```python
from build123d import *

# Parameters (mm, degrees)
SKETCH1_R           = 100
BOSS_EXTRUDE1_DEPTH = 30
FILLET2_R           = 10
SKETCH2_R           = 20
SKETCH2_R_2         = 15
BOSS_EXTRUDE2_DEPTH = 50


with BuildPart() as part:
    # Sketch1 → Boss-Extrude1 (new body)
    with BuildSketch(Plane.XY):
        Circle(SKETCH1_R)
        with BuildLine():
            Line((-10.606601718, -10.606601718), (-49.497474683, -49.497474683))
            ThreePointArc((-49.497474683, -49.497474683), (-69.64553071, -7.03562734), (-58.396917549, 38.597927675))
            Line((-58.396917549, 38.597927675), (-10.606601718, -10.606601718))
        make_face(mode=Mode.SUBTRACT)
        with BuildLine():
            ThreePointArc((10.606601718, -10.606601718), (13.858192988, -5.740251485), (15, 0))
            Line((15, 0), (70, 0))
            ThreePointArc((70, 0), (33.601511791, -61.407966954), (-37.741097297, -58.954300732))
            Line((-37.741097297, -58.954300732), (10.606601718, -10.606601718))
        make_face(mode=Mode.SUBTRACT)
        with BuildLine():
            ThreePointArc((0, 15), (-5.740251485, 13.858192988), (-10.606601718, 10.606601718))
            Line((-10.606601718, 10.606601718), (-49.497474683, 49.497474683))
            ThreePointArc((-49.497474683, 49.497474683), (20.152118643, 67.036498374), (68.585712798, 14))
            Line((68.585712798, 14), (0, 15))
        make_face(mode=Mode.SUBTRACT)
    extrude(amount=BOSS_EXTRUDE1_DEPTH)

    # Fillet2
    fillet2_edges = [part.edges().sort_by_distance(p)[0] for p in [
        (-100, 0, 0),
        (-100, 0, 30),
    ]]
    fillet(fillet2_edges, radius=FILLET2_R)

    # Sketch2 → Boss-Extrude2 (add)
    with BuildSketch(Plane(origin=(0, 0, 0), x_dir=(-1, 0, 0), z_dir=(0, 0, -1))):
        Circle(SKETCH2_R)
        Circle(SKETCH2_R_2, mode=Mode.SUBTRACT)
    extrude(amount=-BOSS_EXTRUDE2_DEPTH)


solid = part.part
```
Model file for the job. Use its own axes, mm. A direction names the side the tool comes from. Round coordinates to 2 decimals unless told otherwise and drop trailing zeros. Put each result on its own line as item: value. Start each with the question number.
Item 1: Cut at B-B (y = -45). Give the number of separate pieces and of enclosed holes in the cut face, then the cut area to 3 significant figures.
Item 2: Mould opens along Y. For faces 4 (the face through (-39.46, 19.1, 14.79)), 5 (the face through (-21, 1, 30)), 6 (the face through (95.38, 30.04, 14.93)) say: released by +Y, released by -Y, zero draft, split by the parting line, or undercut.
Item 3: 3-axis set-ups, long thin cutter, end or side, ignore diameter. For faces 1 (the face through (-18.517, -39.73, 14.79)), 2 (the face through (-18.475, -7.66, 30.206)), 3 (the face through (-3, 15, 50)): which of +Z, -Z, +X, -X, +Y, -Y reach the whole face in a straight line?
Item 4: Drop flat-ended pins along their axis: P1, Ø5, axis at x = -10.5, z = 26, coming from the +Y side; P2, Ø8, axis at y = 14, z = 18, coming from the +X side; P3, Ø5, axis at x = -25.5, y = 71.5, coming from the +Z side. Give the stop position or say it passes through.
Item 5: Drill centre lines: line 1 along Y through (x, z) = (0, 34); line 2 along X through (y, z) = (-18, 5.5); line 3 along X through (y, z) = (-14, 7). Where is each one in solid material? Low to high.
Answer block:
1. separate pieces: 3
1. enclosed holes: 0
1. area: 2,680 mm2
2. face 4: undercut
2. face 5: zero draft
2. face 6: split by the parting line
3. face 1: +Z, -Z
3. face 2: +Z
3. face 3: +Z, +X, -X, +Y, -Y
4. P1: y = 98.85
4. P2: x = 99.5
4. P3: z = 30
5. line 1: -20 to -15, 15 to 20
5. line 2: -97.28 to -67.65, -18 to 8.72, 67.65 to 97.28
5. line 3: -98.55 to -68.59, -14.28 to 14.28, 68.59 to 98.55
